Design review of the part built by this model. Coordinates are the model's own, in mm. Face numbers are marked on the shaded views. A direction names the side the tool comes from. Coordinates: 2 decimals unless noted, no trailing zeros. Order: outer loops, then holes, each group sorted by start corner. A loop starts at its lowest first (then second) coordinate and runs counter-clockwise, first axis right, second up. Notation, with made-up numbers: (57.25, -31.75) - (63.25, -31.75) arc R7 cw to (63.25, -26.75) - close; hole circle Ø5 at (14.25, 4.5). An arc over 180 degrees is marked (long way). Write item = value, one per line. Start each with the question number.
```python
from build123d import *

# Parameters (mm, degrees)
F1_DEPTH = 79.248
F3_DEPTH = 67.31
F4_R     = 7.112
F5_DEPTH = 18.796


with BuildPart() as f1:
    # F0 (on Front) → F1 (new body)
    with BuildSketch(Plane.XZ):
        with BuildLine():
            Line((-42.037, 65.024), (-42.037, 0))
            Line((-42.037, 0), (42.037, 0))
            Line((42.037, 0), (42.037, 65.024))
            Line((42.037, 65.024), (32.385, 65.024))
            Line((32.385, 65.024), (32.385, 14.224))
            ThreePointArc((32.385, 14.224), (30.5251280605, 9.7338719395), (26.035, 7.874))
            Line((26.035, 7.874), (-27.813, 7.874))
            ThreePointArc((-27.813, 7.874), (-32.3031280605, 9.7338719395), (-34.163, 14.224))
            Line((-34.163, 14.224), (-34.163, 65.024))
            Line((-34.163, 65.024), (-42.037, 65.024))
        make_face()
    extrude(amount=F1_DEPTH)

    # F2 (on face) → F3 (cut)
    with BuildSketch(Plane.YZ.offset(42.037)):
        with BuildLine():
            ThreePointArc((-62.1700674157, 30.4810903008), (-74.257569859, 35.6076586923), (-79.248, 47.752))
            Line((-79.248, 47.752), (-79.248, 0))
            Line((-79.248, 0), (-56.896, 0))
            Line((-56.896, 0), (-56.896, 25.1474270113))
            ThreePointArc((-56.896, 25.1474270113), (-58.4371622494, 28.8978853564), (-62.1700674157, 30.4810903008))
        make_face()
        with BuildLine():
            Line((-39.624, 54.864), (-61.976, 54.864))
            ThreePointArc((-61.976, 54.864), (-69.088, 47.752), (-61.976, 40.64))
            Line((-61.976, 40.64), (-39.624, 40.64))
            Line((-39.624, 40.64), (-17.272, 40.64))
            ThreePointArc((-17.272, 40.64), (-10.16, 47.752), (-17.272, 54.864))
            Line((-17.272, 54.864), (-39.624, 54.864))
        make_face()
        with BuildLine():
            Line((0, 0), (0, 47.752))
            ThreePointArc((0, 47.752), (-4.990430141, 35.6076586923), (-17.0779325843, 30.4810903008))
            ThreePointArc((-17.0779325843, 30.4810903008), (-20.8108377506, 28.8978853564), (-22.352, 25.1474270113))
            Line((-22.352, 25.1474270113), (-22.352, 0))
            Line((-22.352, 0), (0, 0))
        make_face()
        with BuildLine():
            Line((0, 65.024), (-17.272, 65.024))
            ThreePointArc((-17.272, 65.024), (-5.0588516753, 59.9651483247), (0, 47.752))
            Line((0, 47.752), (0, 65.024))
        make_face()
        with BuildLine():
            ThreePointArc((-79.248, 47.752), (-74.1891483247, 59.9651483247), (-61.976, 65.024))
            Line((-61.976, 65.024), (-79.248, 65.024))
            Line((-79.248, 65.024), (-79.248, 47.752))
        make_face()
    extrude(amount=-F3_DEPTH, mode=Mode.SUBTRACT)

    # F4 (on face) + F1_face (on face) → F5 (cut)
    with BuildSketch(Plane(origin=(-42.037, 0, 0), x_dir=(0, -1, 0), z_dir=(-1, 0, 0))):
        with BuildLine():
            ThreePointArc((22.352, 47.752), (27.4108516753, 59.9651483247), (39.624, 65.024))
            Line((39.624, 65.024), (0, 65.024))
            Line((0, 65.024), (0, 0))
            Line((0, 0), (22.352, 0))
            Line((22.352, 0), (22.352, 47.752))
        make_face()
        with BuildLine():
            ThreePointArc((39.624, 65.024), (51.8371483247, 59.9651483247), (56.896, 47.752))
            Line((56.896, 47.752), (56.896, 0))
            Line((56.896, 0), (79.248, 0))
            Line((79.248, 0), (79.248, 65.024))
            Line((79.248, 65.024), (39.624, 65.024))
        make_face()
        with Locations((39.624, 47.752)):
            Circle(F4_R)
        with Locations((39.624, 28.702)):
            Circle(F4_R)
    with BuildSketch(Plane(origin=(42.037, -39.624, 32.512), x_dir=(0, 1, 0), z_dir=(1, 0, 0))):
        with BuildLine():
            Line((17.272, -32.512), (17.272, -7.3645729887))
            ThreePointArc((17.272, -7.3645729887), (18.8131622494, -3.6141146436), (22.5460674157, -2.0309096992))
            ThreePointArc((22.5460674157, -2.0309096992), (39.6237274227, 15.3370352392), (22.352, 32.512))
            Line((22.352, 32.512), (-22.352, 32.512))
            ThreePointArc((-22.352, 32.512), (-39.6237274227, 15.3370352392), (-22.5460674157, -2.0309096992))
            ThreePointArc((-22.5460674157, -2.0309096992), (-18.8131622494, -3.6141146436), (-17.272, -7.3645729887))
            Line((-17.272, -7.3645729887), (-17.272, -32.512))
            Line((-17.272, -32.512), (17.272, -32.512))
        make_face()
        with BuildLine():
            ThreePointArc((22.352, 22.352), (29.464, 15.24), (22.352, 8.128))
            Line((22.352, 8.128), (-22.352, 8.128))
            ThreePointArc((-22.352, 8.128), (-29.464, 15.24), (-22.352, 22.352))
            Line((-22.352, 22.352), (22.352, 22.352))
        make_face(mode=Mode.SUBTRACT)
    extrude(amount=-F5_DEPTH, dir=(-1, 0, 0), mode=Mode.SUBTRACT)


solid = f1.part
```
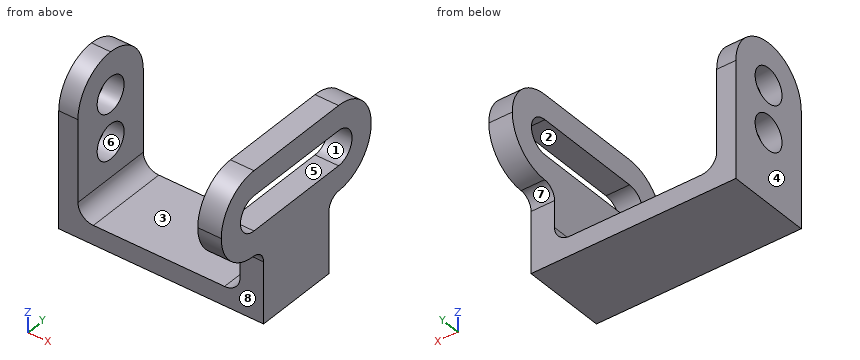
Item 1: For P1, Ø5, axis at x = -20, y = -27, coming from the +Z side; P2, Ø8, axis at x = 27.5, z = 23, coming from the +Y side, all flat-tipped, find the tip position at first contact; note any pin that passes through.
Item 2: For the marked faces 1, 2, 3 and 4, list the 3-axis set-ups (+Z, -Z, +X, -X, +Y, -Y) from which the entire face can be reached by the end or side of a thin tool; tool diameter is ignored.
Item 3: Add section A-A on x = 34. Give the boundary of the cut face in (y, z), plus the area to 3 significant figures.
Item 4: For line 1 (Z direction, x = -37, y = -43); line 2 (X direction, y = -56, z = 26) (3 decimals); line 3 (Z direction, x = 17.5, y = -34), list the stretches that pass through material, from the lowest coordinate up.
Item 5: Add section C-C on z = 46. Give the boundary of the cut face in (x, y) (3 decimals).
Item 6: Add section B-B on y = -25. Give the boundary of the cut face in (x, z) (3 decimals).
Item 7: Add section D-D on z = 38.5. Give the boundary of the cut face in (x, y) (3 decimals).
Item 8: Mouldability with a two-part tool opening along Z and no side actions: class the marked faces 5, 6, 7 and 8 as +Z half, -Z half, draft (parallel to the pull), parting line (faces both ways), or undercut.
Worked out:
q1.P1 = 7.87
q1.P2 = through
q2.face_1 = +X, -X
q2.face_2 = +X
q2.face_3 = +Z, +Y, -Y
q2.face_4 = +Z, -Z, -X, +Y, -Y
q3.outline = (-62.17, 30.48) arc R5.33 cw to (-56.9, 25.15) - (-56.9, 0) - (-22.35, 0) - (-22.35, 25.15) arc R5.33 cw to (-17.08, 30.48) arc R17.27 ccw to (-17.27, 65.02) - (-61.98, 65.02) arc R17.27 ccw to start; hole (-61.98, 40.64) - (-17.27, 40.64) arc R7.11 ccw to (-17.27, 54.86) - (-61.98, 54.86) arc R7.11 ccw to start
q3.area = 2,750 mm2
q4.line_1 = 0 to 22.44, 34.96 to 41.49, 54.01 to 64.69
q4.line_2 = -42.037 to -34.163, 32.385 to 42.037
q4.line_3 = 0 to 7.87
q5.outline = (-42.037, -56.896) - (-34.163, -56.896) - (-34.163, -46.517) - (-42.037, -46.517) - close; (-42.037, -32.731) - (-34.163, -32.731) - (-34.163, -22.352) - (-42.037, -22.352) - close; (32.385, -79.159) - (42.037, -79.159) - (42.037, -68.869) - (32.385, -68.869) - close; (32.385, -10.379) - (42.037, -10.379) - (42.037, -0.089) - (32.385, -0.089) - close
q6.outline = (-42.037, 0) - (42.037, 0) - (42.037, 40.64) - (32.385, 40.64) - (32.385, 14.224) arc R6.35 cw to (26.035, 7.874) - (-27.813, 7.874) arc R6.35 cw to (-34.163, 14.224) - (-34.163, 56.942) - (-42.037, 56.942) - close; (32.385, 54.864) - (42.037, 54.864) - (42.037, 65.024) - (32.385, 65.024) - close
q7.outline = (-42.037, -56.896) - (-34.163, -56.896) - (-34.163, -22.352) - (-42.037, -22.352) - close; (32.385, -76.561) - (42.037, -76.561) - (42.037, -2.687) - (32.385, -2.687) - close
q8.face_5 = undercut
q8.face_6 = undercut
q8.face_7 = -Z half
q8.face_8 = draft
